from build123d import *

# Parameters (mm, degrees)
EXTRUDE_1_DEPTH     = 8
SKETCH_1_3_R        = 10
SKETCH_1_3_R_2      = 4.5
EXTRUDE_2_DEPTH     = 8
SKETCH_2_R          = 8
CUT_EXTRUDE_1_DEPTH = 1.5


with BuildPart() as part:
    # Sketch 1 → Extrude 1 (new body)
    with BuildSketch(Plane(origin=(0, 0, 0), x_dir=(1, 0, 0), z_dir=(0, 1, 0))):
        with BuildLine():
            ThreePointArc((-40.134328358, 5.816588533), (-28.945763891, 9.522165814), (-22, 0))
            ThreePointArc((-22, 0), (-28.945763891, -9.522165814), (-40.134328358, -5.816588533))
            ThreePointArc((-40.134328358, -5.816588533), (-16, -27.712812921), (15.029850746, -37.665642188))
            ThreePointArc((15.029850746, -37.665642188), (9.28068056, -20.306683955), (26, -27.712812921))
            ThreePointArc((26, -27.712812921), (25.773555549, -29.828849769), (25.104477612, -31.849053656))
            ThreePointArc((25.104477612, -31.849053656), (32, 0), (25.104477612, 31.849053656))
            ThreePointArc((25.104477612, 31.849053656), (25.773555549, 29.828849769), (26, 27.712812921))
            ThreePointArc((26, 27.712812921), (9.28068056, 20.306683955), (15.029850746, 37.665642188))
            ThreePointArc((15.029850746, 37.665642188), (-16, 27.712812921), (-40.134328358, 5.816588533))
        make_face()
    extrude(amount=EXTRUDE_1_DEPTH)

    # Sketch 1_3 → Extrude 2 (add)
    # profile 1 of 3: a face of its own
    with BuildSketch(Plane(origin=(0, 0, 0), x_dir=(1, 0, 0), z_dir=(0, 1, 0))):
        with Locations((16, -27.712812921)):
            Circle(SKETCH_1_3_R)
        with Locations(Location((16, -27.712812921, 0), (0, 0, 270))):
            Circle(SKETCH_1_3_R_2, mode=Mode.SUBTRACT)
    # profile 2 of 3: a face of its own
    with BuildSketch(Plane(origin=(0, 0, 0), x_dir=(1, 0, 0), z_dir=(0, 1, 0))):
        with Locations((16, 27.712812921)):
            Circle(SKETCH_1_3_R)
        with Locations(Location((16, 27.712812921, 0), (0, 0, 270))):
            Circle(SKETCH_1_3_R_2, mode=Mode.SUBTRACT)
    # profile 3 of 3: a face of its own
    with BuildSketch(Plane(origin=(0, 0, 0), x_dir=(1, 0, 0), z_dir=(0, 1, 0))):
        with Locations((-32, 0)):
            Circle(SKETCH_1_3_R)
        with Locations(Location((-32, 0, 0), (0, 0, 270))):
            Circle(SKETCH_1_3_R_2, mode=Mode.SUBTRACT)
    extrude(amount=EXTRUDE_2_DEPTH)

    # Sketch 2 → Cut-Extrude 1 (cut)
    with BuildSketch(Plane(origin=(0, 8, 0), x_dir=(1, 0, 0), z_dir=(0, 1, 0))):
        with Locations(Location((-32, 0, 0), (0, 0, 270))):
            Circle(SKETCH_2_R)
        with Locations(Location((16, 27.712812921, 0), (0, 0, 270))):
            Circle(SKETCH_2_R)
        with Locations(Location((16, -27.712812921, 0), (0, 0, 270))):
            Circle(SKETCH_2_R)
    extrude(amount=-CUT_EXTRUDE_1_DEPTH, mode=Mode.SUBTRACT)


solid = part.part
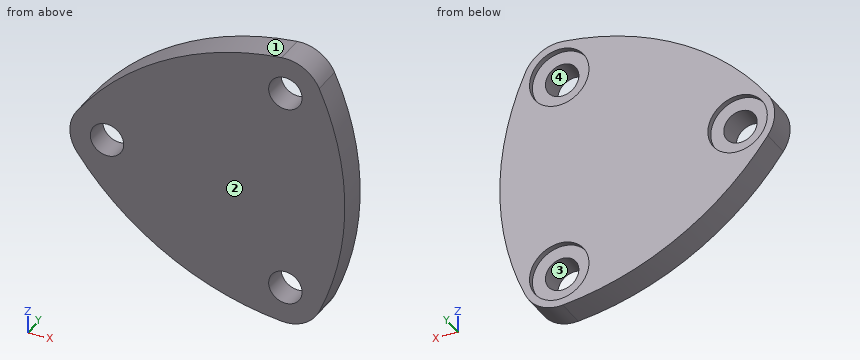
Design review of the part built by this model. Coordinates are the model's own, in mm. Face numbers are marked on the shaded views. Give positions to 0.01 mm unless a question says otherwise; leave off trailing zeros. Order: outer loops, then holes, each group sorted by start corner. A loop starts at its lowest first (then second) coordinate and runs counter-clockwise, first axis right, second up. Notation, with made-up numbers: (-33.5, 81.5) - (16.5, 81.5) arc R16 ccw to (16.5, 92.5) - close; hole circle Ø1 at (-31.75, 54). An arc over 180 degrees is marked (long way). Write item = value, one per line. Start each with the question number.
Q1. Mouldability with a two-part tool opening along X and no side actions: class the marked faces 1, 2, 3 and 4 as released by +X, released by -X, zero draft, split by the parting line, or undercut.
Q2. To check wall thickness, follow L1, parallel to Z at x = -32, y = 4.5; L2, parallel to Z at x = 11, y = 7.5; L3, parallel to Y at x = -36.5, z = 3. State the ranges of each line that lie inside material, in increasing order. Write a range as from..to.
Q3. We need section B-B on y = 3.25. State the section outline as (x, z) points, plus the area to 3 significant figures.
Q4. Clearance check with flat-ended pins moving along their axes: pin 1 Ø8 at (x, z) = (17.5, -25.5) entering from +Y; pin 2 Ø3 at (y, z) = (5, 5.5) entering from +X; pin 3 Ø2 at (y, z) = (5.5, 20.5) entering from +X. State where each tip first meets the part, or that it passes through.
Q5. We need section A-A on x = 16. State the section outline as (y, z) points.
Q6. We need section D-D on x = -32. State the section outline as (y, z) points.
Q7. We need section C-C on z = 0. State the section outline as (x, y) points, plus the area to 4 significant figures.
Working result:
q1.face_1 = released by -X
q1.face_2 = zero draft
q1.face_3 = undercut
q1.face_4 = undercut
q2.L1 = -15.42..-4.5, 4.5..15.42
q2.L2 = -37.17..-33.96, -21.47..21.47, 33.96..37.17
q2.L3 = 0..6.5
q3.outline = (-40.13, -5.82) arc R77 ccw to (15.03, -37.67) arc R10 ccw to (25.1, -31.85) arc R77 ccw to (25.1, 31.85) arc R10 ccw to (15.03, 37.67) arc R77 ccw to (-40.13, 5.82) arc R10 ccw to start; hole circle Ø9 at (-32, 0); hole circle Ø9 at (16, -27.71); hole circle Ø9 at (16, 27.71)
q3.area = 3,840 mm²
q4.pin_1 = 6.5
q4.pin_2 = 31.9
q4.pin_3 = 29.49
q5.outline = (0, -37.71) - (8, -37.71) - (8, -35.71) - (6.5, -35.71) - (6.5, -32.21) - (0, -32.21) - close; (0, -23.21) - (6.5, -23.21) - (6.5, -19.71) - (8, -19.71) - (8, 19.71) - (6.5, 19.71) - (6.5, 23.21) - (0, 23.21) - close; (0, 32.21) - (6.5, 32.21) - (6.5, 35.71) - (8, 35.71) - (8, 37.71) - (0, 37.71) - close
q6.outline = (0, -15.42) - (8, -15.42) - (8, -8) - (6.5, -8) - (6.5, -4.5) - (0, -4.5) - close; (0, 4.5) - (6.5, 4.5) - (6.5, 8) - (8, 8) - (8, 15.42) - (0, 15.42) - close
q7.outline = (-42, 0) - (-36.5, 0) - (-36.5, 6.5) - (-40, 6.5) - (-40, 8) - (-42, 8) - close; (-27.5, 0) - (32, 0) - (32, 8) - (-24, 8) - (-24, 6.5) - (-27.5, 6.5) - close
q7.area = 509.5 mm²
